For this review, use the dimensioned drawing (mm, ordinates from the lowest corner) and the shaded views. A direction names the side the tool comes from. Coordinates: 2 decimals unless noted, no trailing zeros. Write each loop counter-clockwise with the first axis right and the second up, starting at its lowest first coordinate (ties: lowest second). Pieces come first, ordered by that corner, then holes. Notation, with made-up numbers: (74.25, 11.25) -> (119.25, 11.25) arc R25 ccw to (119.25, 36.25) -> close; hole circle Ø6 at (61.5, -21). An arc over 180 degrees is marked (long way). Return JSON: item names as keys, results as strings. Group by question number.
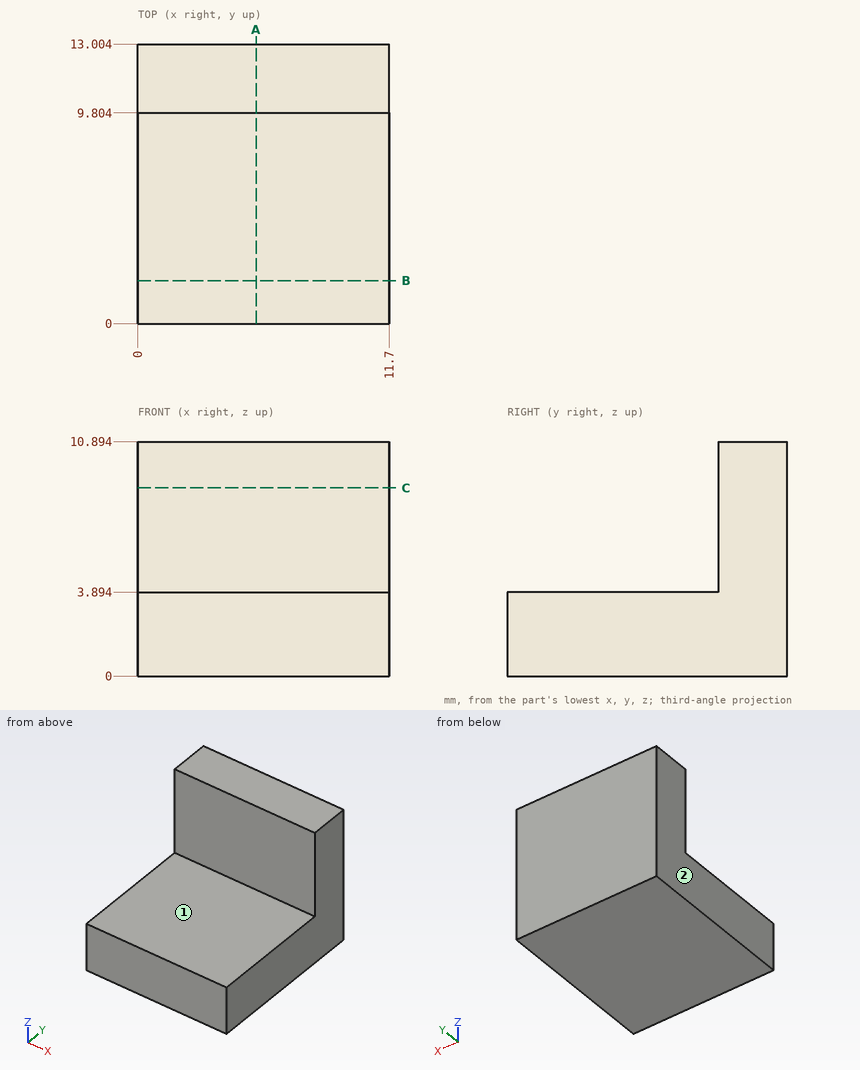
Q1. We need section A-A on x = 5.5. Write out the cut boundary in (y, z) (1 decimal).
Q2. Wall thickness on L1, parallel to Y at x = 6.25, z = 7.5 (1 decimal); L2, parallel to Z at x = 1.5, y = 2.25: over which ranges is each line inside the solid? List them lowest first.
Q3. We need section B-B on y = 2. Write out the cut boundary in (x, z).
Q4. We need section C-C on z = 8.75. Write out the cut boundary in (x, y) (1 decimal).
Q5. For the marked faces 1 and 2, list the 3-axis set-ups (+Z, -Z, +X, -X, +Y, -Y) from which the entire face can be reached by the end or side of a thin tool; tool diameter is ignored.
Q6. For P1, Ø2, axis at x = 10, z = 8, coming from the -Y side; P2, Ø3, axis at x = 3.5, y = 6.5, coming from the +Z side, all flat-tipped, find the tip position at first contact; note any pin that passes through.
Findings below:
{
 "1": {"outline": "(0, 0) -> (13, 0) -> (13, 10.9) -> (9.8, 10.9) -> (9.8, 3.9) -> (0, 3.9) -> close"},
 "2": {"L1": "y = 9.8 to 13", "L2": "z = 0 to 3.89"},
 "3": {"outline": "(0, 0) -> (11.7, 0) -> (11.7, 3.89) -> (0, 3.89) -> close"},
 "4": {"outline": "(0, 9.8) -> (11.7, 9.8) -> (11.7, 13) -> (0, 13) -> close"},
 "5": {"face 1": "+Z, +X, -X, -Y", "face 2": "+Z, -Z, -X, +Y, -Y"},
 "6": {"P1": "stops at y = 9.8", "P2": "stops at z = 3.89"}
}
